Part model, mm, in its own coordinate system. A direction names the side the tool comes from. Coordinates: 2 decimals unless noted, no trailing zeros. Loops run counter-clockwise (first coordinate to the right, second up) from the corner with the lowest first, then second, coordinate; pieces in that order, holes last.
```python
from build123d import *

# Parameters (mm, degrees)
BOSS_EXTRUDE1_DEPTH = 5
FILLET1_R           = 3
FILLET2_R           = 10
FILLET3_R           = 3


with BuildPart() as part:
    # Sketch1 → Revolve1 (revolve)
    with BuildSketch(Plane.XY, mode=Mode.PRIVATE) as revolve1_sk:
        with BuildLine():
            Line((0, 0), (-15, 0))
            Line((-15, 0), (-15, 3))
            Line((-15, 3), (-13, 5))
            ThreePointArc((-13, 5), (-13.688325627, 10.216881481), (-10, 13.97))
            Line((-10, 13.97), (-10, 14.97))
            ThreePointArc((-10, 14.97), (-9.414213562, 16.384213562), (-8, 16.97))
            Line((-8, 16.97), (0, 16.97))
            Line((0, 16.97), (0, 0))
        make_face()
    revolve(revolve1_sk.sketch.rotate(Axis((0, 0, 0), (0, 1, 0)), 270), axis=Axis((0, 0, 0), (0, 1, 0)))

    # Sketch2 → Boss-Extrude1 (add, symmetric)
    with BuildSketch(Plane.XY):
        with BuildLine():
            Line((-6.61, 16.97), (6.61, 16.97))
            ThreePointArc((6.61, 16.97), (7.232167752, 20.609337277), (8.67, 24.01))
            ThreePointArc((8.67, 24.01), (10.247857058, 31.593597712), (7.12, 38.68))
            Line((7.12, 38.68), (0, 46.35))
            Line((0, 46.35), (-1, 50.32))
            Line((-1, 50.32), (0.78, 52.81))
            Line((0.78, 52.81), (12.3, 51.87))
            Line((12.3, 51.87), (14.14, 55.62))
            Line((14.14, 55.62), (3.08, 62.88))
            Line((3.08, 62.88), (4.18, 64.56))
            Line((4.18, 64.56), (0, 67.29))
            Line((0, 67.29), (-1.295560409, 75))
            ThreePointArc((-1.295560409, 75), (-13.70107173, 50.765884766), (-8.67, 24.01))
            ThreePointArc((-8.67, 24.01), (-7.232167752, 20.609337277), (-6.61, 16.97))
        make_face()
    extrude(amount=BOSS_EXTRUDE1_DEPTH, both=True)

    # Fillet1
    fillet1_edges = [part.edges().sort_by_distance(p)[0] for p in [
        (0, 67.29, 0),
    ]]
    fillet(fillet1_edges, radius=FILLET1_R)

    # Fillet2
    # the kernel refuses this fillet: 10 mm, written as the material it adds along each edge
    with BuildSketch(Plane(origin=(-1, 50.32, -5), x_dir=(0.5815472036077696, 0.8135126612265992, 0), z_dir=(0, 0, 1))) as fillet2_piece_1:
        with BuildLine():
            CenterArc((4.753344766, -9.855723924), FILLET2_R, 99.744472398, 39.953038391)
            Line((-2.873057527, -3.387494795), (0, 0))
            Line((0, 0), (3.060800549, 0))
        make_face()
    extrude(amount=10)
    with BuildSketch(Plane(origin=(0, 46.35, -5), x_dir=(-0.24425942618290672, 0.9697099219461441, 0), z_dir=(0, 0, 1))) as fillet2_piece_2:
        with BuildLine():
            CenterArc((FILLET2_R * 0.256126103546, -FILLET2_R), FILLET2_R, 90, 28.732234305)
            Line((-FILLET2_R * 0.224590795698, -FILLET2_R * 0.123124146312), (0, 0))
            Line((0, 0), (FILLET2_R * 0.256126103546, 0))
        make_face()
    extrude(amount=10)
    # the kernel refuses this fillet: 10 mm, written as the material it takes off along each edge
    with BuildSketch(Plane(origin=(7.12, 38.68, -5.825464024), x_dir=(-0.6803411396995018, 0.7328955816706653, 0), z_dir=(0, 0, 1))) as fillet2_2_piece_1:
        with BuildLine():
            CenterArc((0.151797952, 10), FILLET2_R, 267.238538955, 2.761461045)
            ThreePointArc((-0.32998135, 0.011612307), (-0.165028474, 0.004732024), (0, 0))
            Line((0, 0), (0.151797952, 0))
        make_face()
    extrude(amount=11.650928049, mode=Mode.SUBTRACT)

    # Fillet3
    # the kernel refuses this fillet: 3 mm, written as the material it takes off along each edge
    with BuildSketch(Plane(origin=(4.18, 64.56, -12.08398788), x_dir=(-0.5477859413637723, -0.8366185286283144, 0), z_dir=(0, 0, 1))) as fillet3_piece_1:
        with BuildLine():
            CenterArc((3.003276632, -2.830122074), FILLET3_R, 109.373873229, 70.692421457)
            Line((0.00327864, -2.833593255), (-0.056721319, -2.833662679))
            Line((-0.056721319, -2.833662679), (-0.05999996, -6.9424e-05))
            Line((-0.05999996, -6.9424e-05), (0, 0.06))
            ThreePointArc((0, 0.06), (1.004041832, 0.06), (1.988179804, 0.056602441))
            Line((1.988179804, 0.056602441), (2.008083664, 0))
        make_face()
    extrude(amount=24.16797576, mode=Mode.SUBTRACT)


solid = part.part
```
Q1. Mould opens along Y. For faces 6 (the cylindrical face through (-0.66, 1.521, 14.985)), 7 (the cylindrical face through (9.76, 14.48, 2.17)), 8 (the flat face through (0, 16.97, -6)) say: released by +Y, released by -Y, zero draft, split by the parting line, or undercut.
Q2. Tool access for faces 1 (the cylindrical face through (-0.06, 50.23, -0.07)), 2 (the flat face through (0, 44, 5)), 3 (the cylindrical face through (-7.247, 20.659, 0.07)), 4 (the flat face through (-0.75, 71.75, 0.07)), 5 (the cylindrical face through (0.64, 45.9, -0.07)): list every direction of +Z, -Z, +X, -X, +Y, -Y with a clear straight run to the whole face (end or side of a thin tool).
Q3. Saw through at B-B (y = 56.5). List the corners of the cut face in (x, z).
Q4. Saw through at A-A (z = 0). List the corners of the cut face in (x, y).
Q5. Probe line 1 (Z direction, x = -10.25, y = 55); line 2 (Y direction, x = 2, z = 3); line 3 (Y direction, x = 1.75, z = 4.25). List the from-to ranges inside material, lowest first.
Q6. Drop flat-ended pins along their axis: P1, Ø1.5, axis at x = 7.5, z = -1.5, coming from the +Y side; P2, Ø1.5, axis at x = -7, z = -0.5, coming from the +Y side; P3, Ø1.5, axis at x = 1.5, z = -7, coming from the +Y side. Give the stop position or say it passes through.
Checked values:
1. face 6: zero draft
1. face 7: undercut
1. face 8: released by +Y
2. face 1: +Z, -Z
2. face 2: +Z, +X, -X, +Y
2. face 3: +Z, -Z, -X
2. face 4: +Z, -Z, +X, +Y
2. face 5: +Z, -Z, +X
3. outline: (-12.46, -5) - (12.8, -5) - (12.8, 5) - (-12.46, 5) - close
4. outline: (-15, 0) - (15, 0) - (15, 3) - (13, 5) arc R6 ccw to (10, 13.97) - (10, 14.97) arc R2 ccw to (8, 16.97) - (6.61, 16.97) arc R16.04 cw to (8.67, 24.01) arc R12.68 ccw to (7.34, 38.43) arc R10 ccw to (7.02, 38.79) - (1.74, 44.47) arc R10 cw to (-0.17, 47.45) arc R10 cw to (0.78, 52.81) - (12.3, 51.87) - (14.14, 55.62) - (3.08, 62.88) arc R3 ccw to (1.81, 66.11) - (1.1, 66.57) arc R3 cw to (-0.22, 68.59) - (-1.3, 75) arc R42.07 ccw to (-8.67, 24.01) arc R16.04 cw to (-6.61, 16.97) - (-8, 16.97) arc R2 ccw to (-10, 14.97) - (-10, 13.97) arc R6 ccw to (-13, 5) - (-15, 3) - close
5. line 1: z = -5 to 5
5. line 2: y = 0 to 44.2, 52.71 to 65.97
5. line 3: y = 0 to 44.46, 52.73 to 66.15
6. P1: stops at y = 60.47
6. P2: stops at y = 69.26
6. P3: stops at y = 16.97
